```python
from build123d import *

# Parameters (mm, degrees)
SKETCH005_R     = 47.5
PAD002_DEPTH    = 10
SKETCH006_R     = 46.5
POCKET001_DEPTH = 3.5
SKETCH007_R     = 45
PAD003_DEPTH    = 3.5
POCKET003_DEPTH = 10
SKETCH011_W     = 25
SKETCH011_H     = 10
POCKET004_DEPTH = 10
SKETCH014_R     = 2
POCKET007_DEPTH = 10
SKETCH018_W     = 13.2
SKETCH018_H     = 7
POCKET011_DEPTH = 12.5
SKETCH019_W     = 6.5
SKETCH019_H     = 7
POCKET012_DEPTH = 5
SKETCH020_W     = 13.2
SKETCH020_H     = 2.5
PAD005_DEPTH    = 1


with BuildPart() as part:
    # Sketch005 → Pad002 (new body)
    with BuildSketch(Plane.XY):
        Circle(SKETCH005_R)
    extrude(amount=PAD002_DEPTH)

    # Sketch006 (on Face3 of Pad002) → Pocket001 (cut)
    with BuildSketch(Plane.XY.offset(10)):
        Circle(SKETCH006_R)
    extrude(amount=-POCKET001_DEPTH, mode=Mode.SUBTRACT)

    # Sketch007 (on Face5 of Pocket001) → Pad003 (join)
    with BuildSketch(Plane.XY.offset(6.5)):
        Circle(SKETCH007_R)
    extrude(amount=PAD003_DEPTH)

    # Sketch010 (on Face7 of Pad003) → Pocket003 (cut)
    with BuildSketch(Plane.XY.offset(10)):
        Polygon((20, 0), (20, -35), (-20, -35), (-20, 0), (-24, 0), (-24, 30), (24, 30), (24, 0), align=None)
    extrude(amount=-POCKET003_DEPTH, mode=Mode.SUBTRACT)

    # Sketch011 (on Face13 of Pocket003) → Pocket004 (cut)
    with BuildSketch(Plane.XY.offset(10)):
        with Locations((32.5, 0)):
            Rectangle(SKETCH011_W, SKETCH011_H)
    extrude(amount=-POCKET004_DEPTH, mode=Mode.SUBTRACT)

    # Sketch014 (on Face15 of Pocket004) → Pocket007 (cut)
    with BuildSketch(Plane.XY.offset(10)):
        with Locations((-40, 0)):
            Circle(SKETCH014_R)
        with Locations((-12.363995, 38.041183)):
            Circle(SKETCH014_R)
        with Locations((32.356581, 23.51705)):
            Circle(SKETCH014_R)
        with Locations((32.366826, -23.502949)):
            Circle(SKETCH014_R)
        with Locations((-12.347418, -38.046567)):
            Circle(SKETCH014_R)
    extrude(amount=-POCKET007_DEPTH, mode=Mode.SUBTRACT)

    # Sketch018 (on Face9 of Pocket007) → Pocket011 (cut)
    with BuildSketch(Plane.XZ.offset(-30)):
        with Locations((0, 3.5)):
            Rectangle(SKETCH018_W, SKETCH018_H)
    extrude(amount=-POCKET011_DEPTH, mode=Mode.SUBTRACT)

    # Sketch019 (on Face18 of Pocket011) → Pocket012 (cut)
    with BuildSketch(Plane.XZ.offset(-42.5)):
        with Locations((0, 3.5)):
            Rectangle(SKETCH019_W, SKETCH019_H)
    extrude(amount=-POCKET012_DEPTH, mode=Mode.SUBTRACT)

    # Sketch020 (on Face29 of Pocket012) → Pad005 (join)
    with BuildSketch(Plane(origin=(0, 0, 7), x_dir=(1, 0, 0), z_dir=(0, 0, -1))):
        with Locations((0, -34.25)):
            Rectangle(SKETCH020_W, SKETCH020_H)
    extrude(amount=PAD005_DEPTH)


with BuildPart() as part_1:
    # Body002 placement: moved
    add(part.part.moved(Location((0, 0, 5))))


solid = part_1.part
```
Source: CAD feature listing. Evaluate the final solid. Frame: model axes, mm. A direction names the side the tool comes from. Coordinates: 2 decimals unless noted, no trailing zeros. Loops run counter-clockwise (first coordinate to the right, second up) from the corner with the lowest first, then second, coordinate; pieces in that order, holes last. Notation, with made-up numbers: M -37.75,39.25 L 2.25,39.25 A31 ccw 2.25,64.25 Z; hole C 48,-16 d10. An arc over 180 degrees is marked long. Use CSV: the item, a comma, the result in double quotes.
(1) Cut plane B-B on y = -16. Return loops of the section in (x, z).
Answers follow:
outline,"M -44.72,5 L -20,5 L -20,15 L -42.06,15 L -42.06,11.5 L -43.66,11.5 L -43.66,15 L -44.72,15 Z; M 20,5 L 44.72,5 L 44.72,15 L 43.66,15 L 43.66,11.5 L 42.06,11.5 L 42.06,15 L 20,15 Z"
(2) Line query: line 1 (Y direction, x = 0, z = 12.6); line 2 (Y direction, x = 10, z = 13); line 3 (X direction, y = -17, z = 14.25). Output: solid intervals per line, ascending. Write a range as [from, to].
Answers follow:
line 1,"[-47.5, -46.5], [-45, -35], [30, 45], [46.5, 47.5]"
line 2,"[-46.44, -45.41], [-43.87, -35], [30, 43.87], [45.41, 46.44]"
line 3,"[-44.35, -43.28], [-41.67, -20], [20, 41.67], [43.28, 44.35]"
(3) Draft query along X for faces 6 (the face through (34, 5, 10)), 7 (the face through (31, -35, 15)), 8 (the face through (-10.3, -46.37, 9.93)). Return one class per face: pulls with the +X half, pulls with the -X half, needs draft (parallel to the pull), parting line crosses it, or undercut.
Answers follow:
face 6,"undercut"
face 7,"needs draft"
face 8,"parting line crosses it"
(4) Cut plane C-C on x = -40. Return loops of the section in (y, z).
Answers follow:
outline,"M -25.62,5 L -2,5 L -2,15 L -20.62,15 L -20.62,11.5 L -23.71,11.5 L -23.71,15 L -25.62,15 Z; M 2,5 L 25.62,5 L 25.62,15 L 23.71,15 L 23.71,11.5 L 20.62,11.5 L 20.62,15 L 2,15 Z"
(5) Reachability of faces 1 (the face through (20, -20, 10)), 2 (the face through (44.35, 13.97, 13.27)), 3 (the face through (20.4, -9.9, 5)), 4 (the face through (-3.25, 45, 8)), 5 (the face through (0, 34, 11)) from +Z, -Z, +X, -X, +Y, -Y: full face, straight path, thin tool, end or side. Return the list, or none.
Answers follow:
face 1,"+Z, -Z"
face 2,"+Z"
face 3,"-Z, +X, -X, +Y, -Y"
face 4,"-Z, +Y"
face 5,"-Z"
(6) Cut plane A-A on x = 0. Return loops of the section in (y, z).
Answers follow:
outline,"M -47.5,5 L -35,5 L -35,15 L -45,15 L -45,11.5 L -46.5,11.5 L -46.5,15 L -47.5,15 Z; M 30,12 L 33,12 L 33,11 L 35.5,11 L 35.5,12 L 45,12 L 45,15 L 30,15 Z; M 46.5,12 L 47.5,12 L 47.5,15 L 46.5,15 Z"
(7) Cut plane D-D on z = 9.5. Return loops of the section in (x, y).
Answers follow:
outline,"M -24,0 L -24,30 L -6.6,30 L -6.6,42.5 L -3.25,42.5 L -3.25,47.39 A47.5 ccw long 3.25,47.39 L 3.25,42.5 L 6.6,42.5 L 6.6,30 L 24,30 L 24,5 L 45,5 L 45,-5 L 20,-5 L 20,-35 L -20,-35 L -20,0 Z; hole C -40,0 d4; hole C -12.36,38.04 d4; hole C -12.35,-38.05 d4; hole C 32.36,23.52 d4; hole C 32.37,-23.5 d4"
(8) Contact query for flat-ended pins moving along their axis: pin 1 (1.5 mm diameter, centred on y = 44.5, z = 7.5, fed in from -X); pin 2 (5.5 mm diameter, centred on y = 37.5, z = 7, fed in from +X); pin 3 (2 mm diameter, centred on x = -14, z = 7.5, fed in from -Y). Output: stop coordinate, or through.
Answers follow:
pin 1,"x = -18.5"
pin 2,"x = 32.38"
pin 3,"y = -45.69"
